Input: part model. Units: mm. Frame: model coordinates. A direction names the side the tool comes from. Round coordinates to 2 decimals unless told otherwise and drop trailing zeros. Order: outer loops, then holes, each group sorted by start corner. A loop starts at its lowest first (then second) coordinate and runs counter-clockwise, first axis right, second up.
Item 1: Cut plane A-A on z = 15.5. Output: boundary loops of the cut face in (x, y), then the cut area to 3 significant figures.
Item 2: Mould query, pull axis Y, two halves, no side actions, for faces 4 (the flat face through (-2.493, 5, 41)), 5 (the cylindrical face through (14.307, 4.506, 17.042)), 6 (the flat face through (-2, -3, 15)), 7 (the cylindrical face through (-5.158, 3.955, 7.902)). Classes: released by +Y, released by -Y, zero draft, split by the parting line, or undercut.
Item 3: Reachability of faces 1 (the flat face through (-5, 0, 40)), 2 (the flat face through (-6.3, 10.4, 30)), 3 (the flat face through (4, 0, 42)) from +Z, -Z, +X, -X, +Y, -Y: full face, straight path, thin tool, end or side. Return the list, or none.
Item 4: First-contact query: pin 1 (1 mm diameter, centred on y = -4, z = 11.5, fed in from +X); pin 2 (10 mm diameter, centred on y = 10.5, z = 6.5, fed in from +X); pin 3 (8 mm diameter, centred on y = -8, z = 4.5, fed in from +X). Flat tips, straight axial feed; report the tip coordinate or a pass-through.
Item 5: Line query: L1, parallel to Y at x = 0, z = 31.5; L2, parallel to X at y = 0, z = 11; L3, parallel to X at y = 2.5, z = 38.5. Output: solid intervals per line, ascending.
Item 6: Cut plane B-B on z = 36.5. Output: boundary loops of the cut face in (x, y), then the cut area to 3 significant figures.
```python
from build123d import *

# Parameters (mm, degrees)
F0_R           = 15
F1_DEPTH       = 30
F2_R           = 12
F3_DEPTH       = 2
F5_DEPTH       = 10
F6_DEPTH       = 8
F7_D           = 6.5
F7_CBORE_D     = 13
F7_CBORE_DEPTH = 15
F8_SIZE        = 5
F9_R           = 1


with BuildPart() as f1:
    # F0 (on Top) → F1 (new body)
    with BuildSketch(Plane.XY):
        Circle(F0_R)
    extrude(amount=F1_DEPTH)

    # F2 (on face) → F3 (join)
    with BuildSketch(Plane.XY.offset(30)):
        Circle(F2_R)
    extrude(amount=F3_DEPTH)

    # F4 (on face) → F5 (join)
    with BuildSketch(Plane.XY.offset(32)):
        with BuildLine():
            ThreePointArc((-2.492736493, -8.6479052248), (5.411347871, -7.1914751073), (9, 0))
            ThreePointArc((9, 0), (5.411347871, 7.1914751073), (-2.492736493, 8.6479052248))
            Line((-2.492736493, 8.6479052248), (-2.492736493, -8.6479052248))
        make_face()
    extrude(amount=F5_DEPTH)

    # F4 (on face) → F6 (join)
    with BuildSketch(Plane.XY.offset(32)):
        with BuildLine():
            Line((-2.492736493, -8.6479052248), (-2.492736493, 8.6479052248))
            ThreePointArc((-2.492736493, 8.6479052248), (-9, 0), (-2.492736493, -8.6479052248))
        make_face()
    extrude(amount=F6_DEPTH)

    # F7 (through all)
    with Locations(Plane(origin=(0, 0, 0), x_dir=(1, 0, 0), z_dir=(0, 0, -1))):
        with Locations((0, 0)):
            CounterBoreHole(F7_D / 2, F7_CBORE_D / 2, F7_CBORE_DEPTH)

    # F8
    f8_edges = [f1.edges().sort_by_distance(p)[0] for p in [
        (-15, 0, 0),
    ]]
    chamfer(f8_edges, length=F8_SIZE)

    # F9
    f9_edges = [f1.edges().sort_by_distance(p)[0] for p in [
        (-15, 0, 30),
        (-10, 0, 0),
        (-15, 0, 5),
        (-6.5, 0, 0),
    ]]
    fillet(f9_edges, radius=F9_R)


solid = f1.part
```
From the geometry:
1. outline: circle Ø30 at (0, 0); hole circle Ø6.5 at (0, 0)
1. area: 674 mm2
2. face 4: zero draft
2. face 5: split by the parting line
2. face 6: undercut
2. face 7: undercut
3. face 1: +Z, -X, +Y, -Y
3. face 2: +Z
3. face 3: +Z, +X, -X, +Y, -Y
4. pin 1: stops at x = 14.59
4. pin 2: stops at x = 13.96
4. pin 3: stops at x = 14.43
5. L1: y = -12 to -3.25, 3.25 to 12
5. L2: x = -15 to -6.5, 6.5 to 15
5. L3: x = -8.65 to -2.08, 2.08 to 8.65
6. outline: circle Ø18 at (0, 0); hole circle Ø6.5 at (0, 0)
6. area: 221 mm2
